For this review, take the finished solid that the model builds, in its own axes (mm). A direction names the side the tool comes from. Round coordinates to 2 decimals unless told otherwise and drop trailing zeros. Loops run counter-clockwise (first coordinate to the right, second up) from the corner with the lowest first, then second, coordinate; pieces in that order, holes last.
1. To check wall thickness, follow line 1 along Y through (x, z) = (0, 8.25) (3 decimals); line 2 along Z through (x, y) = (-32.5, -0.5) (3 decimals); line 3 along Z through (x, y) = (-2.5, 5) (3 decimals). State the ranges of each line that lie inside material, in increasing order.
2. Draft analysis for pull direction Y (two halves, no side actions). For faces 4 (the flat face through (8, -16, 0)), 5 (the flat face through (0, 0, 3.175)), 6 (the cylindrical face through (3.441, -15.497, 8.81)), 7 (the cylindrical face through (-2.75, -12.4, 9.61)), state which applies: released by +Y, released by -Y, zero draft, split by the parting line, or undercut.
3. Clearance check with flat-ended pins moving along their axes: pin 1 Ø8 at (x, y) = (-20.5, -27.5) entering from +Z (3 decimals); pin 2 Ø1 at (x, y) = (-18.5, -20) entering from -Z; pin 3 Ø2 at (x, z) = (14, 3.5) entering from -Y. State where each tip first meets the part, or that it passes through.
4. Consider section A-A on x = 0. State the section outline as (y, z) points (1 decimal), then the cut area to 3 significant figures.
5. Tool access review of faces 1 (the cylindrical face through (34.826, 10.967, 0.313)), 2 (the flat face through (15, -7, 3.175)), 3 (the cylindrical face through (3.441, -15.497, -20.349)): name each direction out of +Z, -Z, +X, -X, +Y, -Y from which nothing blocks a thin tool from reaching the whole face with its end or side.
6. Consider section D-D on z = 8.5. State the section outline as (x, y) points (3 decimals).
7. Consider section C-C on z = -24. State the section outline as (x, y) points (3 decimals), then the cut area to 3 significant figures.
from build123d import *

# Parameters (mm, degrees)
SKETCH1_R           = 36.5125
BOSS_EXTRUDE1_DEPTH = 3.175
SKETCH2_R           = 15.875
BOSS_EXTRUDE2_DEPTH = 41.275
SKETCH2_2_R         = 15.875
BOSS_EXTRUDE3_DEPTH = 15.875
SKETCH3_R           = 12.7
CUT_EXTRUDE1_DEPTH  = 12.7
FILLET1_R           = 2.54
FILLET2_R           = 1.27


with BuildPart() as part:
    # Sketch1 → Boss-Extrude1 (new body)
    with BuildSketch(Plane.XY):
        Circle(SKETCH1_R)
    extrude(amount=BOSS_EXTRUDE1_DEPTH)

    # Sketch2 → Boss-Extrude2 (add)
    with BuildSketch(Plane(origin=(0, 0, 0), x_dir=(-1, 0, 0), z_dir=(0, 0, -1))):
        Circle(SKETCH2_R)
    extrude(amount=BOSS_EXTRUDE2_DEPTH)

    # Sketch2_2 → Boss-Extrude3 (add)
    with BuildSketch(Plane(origin=(0, 0, 0), x_dir=(-1, 0, 0), z_dir=(0, 0, -1))):
        Circle(SKETCH2_2_R)
    extrude(amount=-BOSS_EXTRUDE3_DEPTH)

    # Sketch3 → Cut-Extrude1 (cut)
    with BuildSketch(Plane.XY.offset(15.875)):
        Circle(SKETCH3_R)
    extrude(amount=-CUT_EXTRUDE1_DEPTH, mode=Mode.SUBTRACT)

    # Fillet1
    fillet1_edges = [part.edges().sort_by_distance(p)[0] for p in [
        (-36.5125, 0, 3.175),
    ]]
    fillet(fillet1_edges, radius=FILLET1_R)

    # Fillet2
    fillet2_edges = [part.edges().sort_by_distance(p)[0] for p in [
        (15.875, 0, 15.875),
    ]]
    fillet(fillet2_edges, radius=FILLET2_R)


solid = part.part
Resolved:
1. line 1: y = -15.875 to -12.7, 12.7 to 15.875
1. line 2: z = 0 to 3.175
1. line 3: z = -41.275 to 3.175
2. face 4: zero draft
2. face 5: undercut
2. face 6: split by the parting line
2. face 7: undercut
3. pin 1: stops at z = 3.175
3. pin 2: stops at z = 0
3. pin 3: stops at y = -32.91
4. outline: (-36.5, 0) - (-15.9, 0) - (-15.9, -41.3) - (15.9, -41.3) - (15.9, 0) - (36.5, 0) - (36.5, 0.6) arc R2.5 ccw to (34, 3.2) - (15.9, 3.2) - (15.9, 14.6) arc R1.3 ccw to (14.6, 15.9) - (12.7, 15.9) - (12.7, 3.2) - (-12.7, 3.2) - (-12.7, 15.9) - (-14.6, 15.9) arc R1.3 ccw to (-15.9, 14.6) - (-15.9, 3.2) - (-34, 3.2) arc R2.5 ccw to (-36.5, 0.6) - close
4. area: 1,620 mm2
5. face 1: +Z, -Z
5. face 2: +Z
5. face 3: -Z
6. outline: circle Ø31.75 at (0, 0); hole circle Ø25.4 at (0, 0)
7. outline: circle Ø31.75 at (0, 0)
7. area: 792 mm2
